Source: CAD feature listing. Evaluate the final solid. Frame: model axes, mm. A direction names the side the tool comes from. Give positions to 0.01 mm unless a question says otherwise; leave off trailing zeros. Loops run counter-clockwise (first coordinate to the right, second up) from the corner with the lowest first, then second, coordinate; pieces in that order, holes last.
Autodesk Fusion 360 part; units mm, degrees
sketch "Skizze1" plane through (0, 0, 0) normal (0, 0, 1) x (1, 0, 0)
  circle A0 centre (0, 0) radius 13.5
  circle A1 centre (0, 0) radius 12
  circle A2 centre (0, 0) radius 2
  dimension "d1" = 27
  dimension "d2" = 24
  dimension "d3" = 4
extrude "Extrusion1" add sketch "Skizze1" along normal blind 10 contours A0
extrude "Extrusion2" add sketch "Skizze1" against normal blind 8 contours A0 | A1
sketch "Skizze2" plane through (0, 0, -8) normal (0, 0, -1) x (1, 0, 0)
  circle A0 centre (0, 0) radius 2
  circle A1 centre (0, 0) radius 13.5
  circle A2 centre (0, 0) radius 13.5
  circle A3 centre (0, 0) radius 11.5
  dimension "d8" = -2
extrude "Extrusion3" cut sketch "Skizze2" against normal blind 2 contours A3
(1) Reachability of faces 1 (the cylindrical face through (-1.5, -11.4, -7)), 2 (the cylindrical face through (-11.99, -0.53, 4.93)), 3 (the cylindrical face through (0, -2, -3)) from +Z, -Z, +X, -X, +Y, -Y: full face, straight path, thin tool, end or side. Return the list, or none.
A:
face 1: -Z
face 2: +Z
face 3: +Z, -Z
(2) Section C-C, the plane z = 8. Return the cut outline in (x, y), then the cut area to 3 significant figures.
A:
outline: circle Ø27 at (0, 0); hole circle Ø24 at (0, 0)
area: 120 mm2
(3) First-contact query: pin 1 (1.5 mm diameter, centred on y = -4.5, z = 5, fed in from +X); pin 2 (3 mm diameter, centred on x = 0, y = 6, fed in from +Z); pin 3 (8 mm diameter, centred on x = 8, z = -5.5, fed in from +Y). Flat tips, straight axial feed; report the tip coordinate or a pass-through.
A:
pin 1: stops at x = 12.97
pin 2: stops at z = 0
pin 3: stops at y = 12.89
(4) Ray query, line 1 along Y through (x, z) = (0, -7.25); line 2 along Y through (x, z) = (0, -3.1); line 3 along Z through (x, y) = (-10.5, -5.5). Return the intervals inside material, ascending.
A:
line 1: y = -13.5 to -11.5, 11.5 to 13.5
line 2: y = -13.5 to -2, 2 to 13.5
line 3: z = -8 to 0
(5) Section A-A, the plane x = 0. Return the cut outline in (y, z), then the cut area to 3 significant figures.
A:
outline: (-13.5, -8) - (-11.5, -8) - (-11.5, -6) - (-2, -6) - (-2, 0) - (-12, 0) - (-12, 10) - (-13.5, 10) - close; (2, -6) - (11.5, -6) - (11.5, -8) - (13.5, -8) - (13.5, 10) - (12, 10) - (12, 0) - (2, 0) - close
area: 176 mm2
(6) Mould query, pull axis X, two halves, no side actions, for faces 4 (the flat face through (-0.2, 2.4, -6)), 5 (the cylindrical face through (-2.93, -13.18, 1.13)), 6 (the flat face through (10, 6, -8)). Classes: pulls with the +X half, pulls with the -X half, needs draft (parallel to the pull), parting line crosses it, or undercut.
A:
face 4: undercut
face 5: parting line crosses it
face 6: needs draft
(7) Section D-D, the plane x = 8. Return the cut outline in (y, z).
A:
outline: (-10.87, -8) - (-8.26, -8) - (-8.26, -6) - (8.26, -6) - (8.26, -8) - (10.87, -8) - (10.87, 10) - (8.94, 10) - (8.94, 0) - (-8.94, 0) - (-8.94, 10) - (-10.87, 10) - close
